from build123d import *

# Parameters (mm, degrees)
SKETCH1_W           = 400
SKETCH1_H           = 420
SKETCH1_W_2         = 380
SKETCH1_H_2         = 400
BOSS_EXTRUDE1_DEPTH = 20
SKETCH2_R           = 3
CUT_EXTRUDE1_DEPTH  = 400
SKETCH3_R           = 3
CUT_EXTRUDE2_DEPTH  = 420


with BuildPart() as part:
    # Sketch1 → Boss-Extrude1 (new body)
    with BuildSketch(Plane(origin=(0, 0, 0), x_dir=(1, 0, 0), z_dir=(0, 1, 0))):
        Rectangle(SKETCH1_W, SKETCH1_H)
        Rectangle(SKETCH1_W_2, SKETCH1_H_2, mode=Mode.SUBTRACT)
    extrude(amount=BOSS_EXTRUDE1_DEPTH)

    # Sketch2 → Cut-Extrude1 (cut)
    with BuildSketch(Plane.ZY.offset(200)):
        with Locations((1.026e-06, 10)):
            Circle(SKETCH2_R)
        with Locations((129.999998686, 10)):
            Circle(SKETCH2_R)
        with Locations((-130, 10)):
            Circle(SKETCH2_R)
    extrude(amount=-CUT_EXTRUDE1_DEPTH, mode=Mode.SUBTRACT)

    # Sketch3 → Cut-Extrude2 (cut)
    with BuildSketch(Plane(origin=(0, 0, -210), x_dir=(-1, 0, 0), z_dir=(0, 0, -1))):
        with Locations((-150, 10)):
            Circle(SKETCH3_R)
        with Locations((150, 10)):
            Circle(SKETCH3_R)
    extrude(amount=-CUT_EXTRUDE2_DEPTH, mode=Mode.SUBTRACT)


solid = part.part
Part model, mm, in its own coordinate system. A direction names the side the tool comes from. Coordinates: 2 decimals unless noted, no trailing zeros. Order: outer loops, then holes, each group sorted by start corner. A loop starts at its lowest first (then second) coordinate and runs counter-clockwise, first axis right, second up. Notation, with made-up numbers: M 0.5,74.25 L 38.5,74.25 A27 ccw 38.5,102.25 Z; hole C 8.25,56 d8. An arc over 180 degrees is marked long. Use a Markdown table: item, result.
(1) Tool access for faces 5 (the flat face through (-3, 10, 200)), 6 (the flat face through (-194, 0, -1)): list every direction of +Z, -Z, +X, -X, +Y, -Y with a clear straight run to the whole face (end or side of a thin tool).
A:
| item | result |
|---|---|
| face 5 | +Y, -Y |
| face 6 | +Z, -Z, +X, -X, -Y |
(2) Cut at A-A on z = 18.5. Write the cut outline in (x, y).
A:
| item | result |
|---|---|
| outline | M -200,0 L -190,0 L -190,20 L -200,20 Z; M 190,0 L 200,0 L 200,20 L 190,20 Z |
(3) Pull direction Z, two halves, no side cores. Call faces 1 (the flat face through (190, 12, 3)), 2 (the flat face through (-3, 10, 210)), 3 (the flat face through (-3, 10, -210)), 4 (the flat face through (-3, 10, -200)): released by +Z, released by -Z, zero draft, split by the parting line, or undercut.
A:
| item | result |
|---|---|
| face 1 | undercut |
| face 2 | released by +Z |
| face 3 | released by -Z |
| face 4 | undercut |
(4) Cut at C-C on x = 173. Write the cut outline in (y, z), then the cut area to 3 significant figures.
A:
| item | result |
|---|---|
| outline | M 0,-210 L 20,-210 L 20,-200 L 0,-200 Z; M 0,200 L 20,200 L 20,210 L 0,210 Z |
| area | 400 mm^2 |
(5) Cut at B-B on y = 16.5. Write the cut outline in (x, z).
A:
| item | result |
|---|---|
| outline | M -200,-210 L 200,-210 L 200,210 L -200,210 Z; hole M -190,-200 L 190,-200 L 190,200 L -190,200 Z |
(6) Flat gauge pin, fed straight in: pin 1 (8 mm diameter, centred on y = 10, z = 0, fed in from -X). Where does the tip first touch, or does it go through?
A:
| item | result |
|---|---|
| pin 1 | stops at x = -200 |
(7) Probe L1, parallel to Z at x = 90, y = 6.75; L2, parallel to X at y = 9.25, z = -118; L3, parallel to Y at x = 150, z = -207. List the from-to ranges inside material, lowest first.
A:
| item | result |
|---|---|
| L1 | z = -210 to -200, 200 to 210 |
| L2 | x = -200 to -190, 190 to 200 |
| L3 | y = 0 to 7, 13 to 20 |
